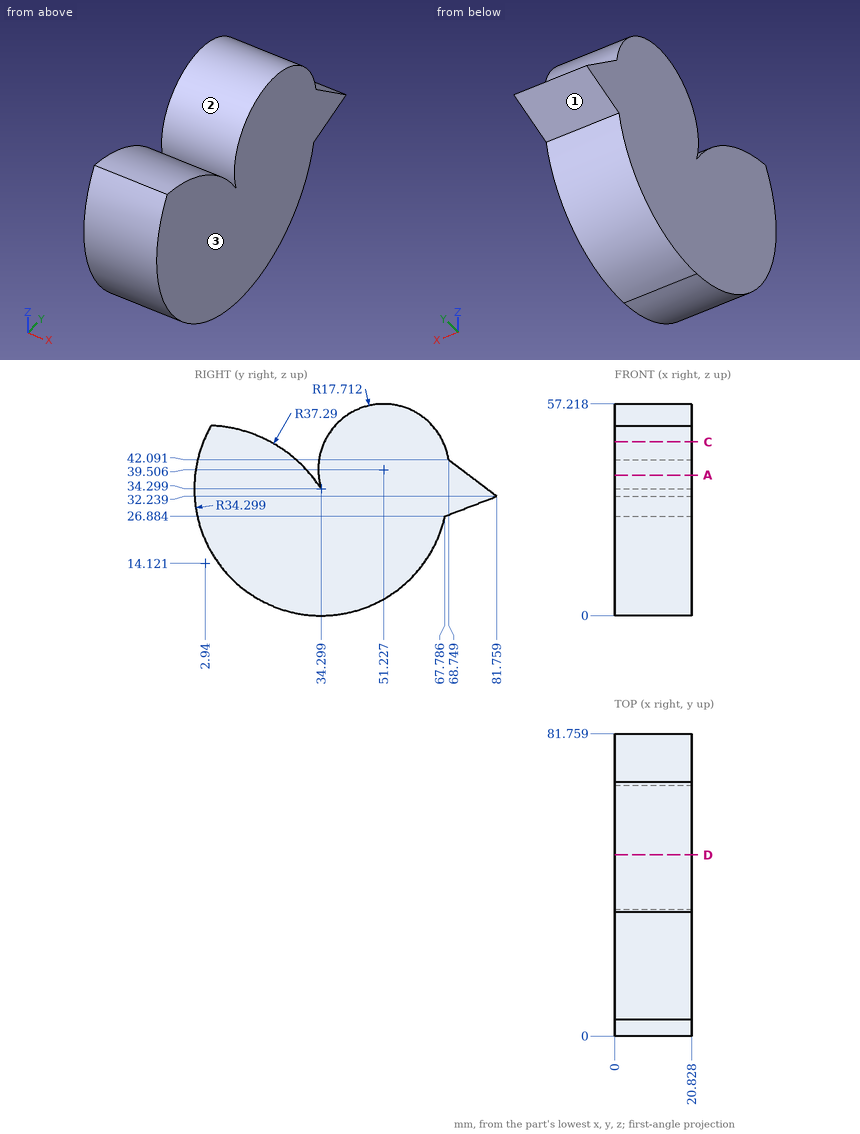
Check sheet for the drawn part. Datum: minimum x, y, z corner. Units: mm. Give positions to 0.01 mm unless a question says otherwise; leave off trailing zeros. Write each loop counter-clockwise with the first axis right and the second up, starting at its lowest first coordinate (ties: lowest second). Pieces come first, ordered by that corner, then holes. Notation, with made-up numbers: M -35,44 L -12,44 A15 ccw -12,49 Z; hole C 55,40.5 d1. An arc over 180 degrees is marked long. One line per question, with ' | ' between items.
1) Gauge pin test, flat ends, axial feed: pin 1 Ø5 at (x, z) = (4, 45) entering from -Y (1 decimal); pin 2 Ø8 at (x, z) = (6.5, 41) entering from +Y; pin 3 Ø3 at (y, z) = (62, 28.5) entering from -X; pin 4 Ø8 at (x, y) = (3.5, 21.5) entering from -Z. Record the tip position at first contact, or that the pin passes through.
Result:
pin 1: stops at y = 1 | pin 2: stops at y = 75.47 | pin 3: stops at x = 0 | pin 4: stops at z = 1.15
2) Thickness scan on line 1 along Y through (x, z) = (2, 43) (1 decimal); line 2 along Y through (x, z) = (9.75, 39) (1 decimal); line 3 along Z through (x, y) = (2.5, 30) (1 decimal). Record the ranges inside material, lowest first. Write a range as [from, to].
Result:
line 1: y = [1.1, 26.5], [33.9, 68.6] | line 2: y = [0.3, 30.7], [33.5, 72.8] | line 3: z = [0.3, 39.8]
3) Section check C-C on z = 47. Enter the section's corners in (x, y) (1 decimal), plus the area to 3 significant figures.
Result:
outline: M 0,2.4 L 20.8,2.4 L 20.8,20.5 L 0,20.5 Z; M 0,35.2 L 20.8,35.2 L 20.8,67.3 L 0,67.3 Z | area: 1,050 mm2
4) Section check D-D on y = 49. Enter the section's corners in (x, z), plus the area to 3 significant figures.
Result:
outline: M 0,3.31 L 20.83,3.31 L 20.83,57.08 L 0,57.08 Z | area: 1,120 mm2
5) Section check A-A on z = 38. Enter the section's corners in (x, y).
Result:
outline: M 0,0.2 L 20.83,0.2 L 20.83,31.58 L 0,31.58 Z; M 0,33.58 L 20.83,33.58 L 20.83,74.15 L 0,74.15 Z
6) Mould release check, pull along Y, two halves, no side actions. Record for the marked faces 1, 2 and 3: released by +Y, released by -Y, zero draft, split by the parting line, or undercut.
Result:
face 1: released by +Y | face 2: undercut | face 3: zero draft
